Here's how the part is built. I have some questions about the finished solid (model axes, mm). Coordinates: 2 decimals unless noted, no trailing zeros. Loops run counter-clockwise (first coordinate to the right, second up) from the corner with the lowest first, then second, coordinate; pieces in that order, holes last. Notation, with made-up numbers: (21, 37) -> (47, 37) arc R12 ccw to (47, 57) -> close; hole circle Ø11 at (21, 83). An arc over 180 degrees is marked (long way). Answer as a JSON object with one key per item and string values. Group by question number.
1) I need wall thicknesses on probe 1 along Y at (x, z) = (0, 4.25) (3 decimals); probe 2 along Y at (x, z) = (1, 10.75) (3 decimals); probe 3 along X at (y, z) = (10.5, 9). Which ranges of each line are inside material? Lowest first, please. Write a range as [from, to].
2) I want a section at B-B (z = 2.75). Write out the boundary of the cut face in (x, y) (3 decimals), then the cut area to 3 significant figures.
3) If we mould it in two halves opening along Y, with no side actions, what happens to faces 1 (the cylindrical face through (0.81, -11.47, 6.18)), 2 (the flat face through (6.096, 0, 6)), 3 (the flat face through (0, -15.875, 6))? For each: +Y half, -Y half, draft (parallel to the pull), parting line (faces both ways), or undercut.
4) I want a section at A-A (x = 0). Write out the boundary of the cut face in (y, z) (3 decimals).
5) I want a section at C-C (x = 1.75). Count the separate pieces of the cut face and the enclosed holes in it, then the cut area to 3 significant figures.
```python
from build123d import *

# Parameters (mm, degrees)
SKETCH1_W                            = 12.192
SKETCH1_H                            = 31.75
BOSS_EXTRUDE1_DEPTH                  = 12.192
FILLET1_R                            = 0.381
F_19_0_166_DIAMETER_HOLE1_AT_2_COUNT = 2
F_19_0_166_DIAMETER_HOLE1_AT_2_PITCH = 19.05


with BuildPart() as part:
    # Sketch1 → Boss-Extrude1 (new body)
    with BuildSketch(Plane.XY):
        Rectangle(SKETCH1_W, SKETCH1_H)
    extrude(amount=BOSS_EXTRUDE1_DEPTH)

    # Fillet1
    fillet1_edges = [part.edges().sort_by_distance(p)[0] for p in [
        (-6.096, 15.875, 6.096),
        (6.096, 15.875, 6.096),
        (6.096, -15.875, 6.096),
        (-6.096, -15.875, 6.096),
    ]]
    fillet(fillet1_edges, radius=FILLET1_R)

    # Sketch2 → #19 (0.166) Diameter Hole1 (revolve, cut)
    with BuildSketch(Plane(origin=(0, 9.525, 12.192), x_dir=(0, -1, 0), z_dir=(1, 0, 0))):
        Polygon((0, 0), (0, 12.192), (2.286, 12.192), (2.1082, 12.0142), (2.1082, 0.1778), (2.286, 0), align=None)
    f_19_0_166_diameter_hole1 = revolve(axis=Axis((0, 9.525, 18.542), (0, 0, -1)), mode=Mode.SUBTRACT)

    # #19 (0.166) Diameter Hole1 at 2: #19 (0.166) Diameter Hole1 ×2
    with Locations(*[(0, -i * F_19_0_166_DIAMETER_HOLE1_AT_2_PITCH, 0) for i in range(1, F_19_0_166_DIAMETER_HOLE1_AT_2_COUNT)]):
        add(f_19_0_166_diameter_hole1, mode=Mode.SUBTRACT)


solid = part.part
```
Determined:
{
 "1": {"probe 1": "[-15.875, -11.633], [-7.417, 7.417], [11.633, 15.875]", "probe 2": "[-15.875, -11.381], [-7.669, 7.669], [11.381, 15.875]", "probe 3": "[-6.1, -1.87], [1.87, 6.1]"},
 "2": {"outline": "(-6.096, -15.494) arc R0.381 ccw to (-5.715, -15.875) -> (5.715, -15.875) arc R0.381 ccw to (6.096, -15.494) -> (6.096, 15.494) arc R0.381 ccw to (5.715, 15.875) -> (-5.715, 15.875) arc R0.381 ccw to (-6.096, 15.494) -> close; hole circle Ø4.216 at (0, -9.525); hole circle Ø4.216 at (0, 9.525)", "area": "359 mm^2"},
 "3": {"face 1": "undercut", "face 2": "draft", "face 3": "-Y half"},
 "4": {"outline": "(-15.875, 0) -> (-11.811, 0) -> (-11.633, 0.178) -> (-11.633, 12.014) -> (-11.811, 12.192) -> (-15.875, 12.192) -> close; (-7.417, 0.178) -> (-7.239, 0) -> (7.239, 0) -> (7.417, 0.178) -> (7.417, 12.014) -> (7.239, 12.192) -> (-7.239, 12.192) -> (-7.417, 12.014) -> close; (11.633, 0.178) -> (11.811, 0) -> (15.875, 0) -> (15.875, 12.192) -> (11.811, 12.192) -> (11.633, 12.014) -> close"},
 "5": {"separate pieces": "3", "enclosed holes": "0", "area": "330 mm^2"}
}
